from build123d import *

# Parameters (mm, degrees)
SCHIZZO2_W                 = 24
SCHIZZO2_H                 = 35
BASESUPPORTO_DEPTH         = 5
SCHIZZO3_R                 = 8
APPOGGIOALLONGHERONE_DEPTH = 31.120590964
SCHIZZO4_W                 = 5
SCHIZZO4_H                 = 3
FORIFASCETTE_DEPTH         = 22.800229357


with BuildPart() as part:
    # Schizzo2 → BaseSupporto (new body)
    with BuildSketch(Plane(origin=(0, 0, 0), x_dir=(1, 0, 0), z_dir=(0, 1, 0))):
        Rectangle(SCHIZZO2_W, SCHIZZO2_H)
    extrude(amount=BASESUPPORTO_DEPTH)

    # Schizzo3 → AppoggioAlLongherone (cut, through all)
    with BuildSketch(Plane.ZY.offset(12)):
        with Locations((-25.099342077, 2.5)):
            Circle(SCHIZZO3_R)
    extrude(amount=-APPOGGIOALLONGHERONE_DEPTH, mode=Mode.SUBTRACT)

    # Schizzo4 → ForiFascette (cut, through all)
    with BuildSketch(Plane(origin=(0, 5, 0), x_dir=(1, 0, 0), z_dir=(0, 1, 0))):
        with Locations((-6, 14)):
            Rectangle(SCHIZZO4_W, SCHIZZO4_H)
        with Locations((6, 14)):
            Rectangle(SCHIZZO4_W, SCHIZZO4_H)
    extrude(amount=-FORIFASCETTE_DEPTH, mode=Mode.SUBTRACT)


solid = part.part
Source: CAD feature listing. Evaluate the final solid. Frame: model axes, mm. A direction names the side the tool comes from. Give positions to 0.01 mm unless a question says otherwise; leave off trailing zeros. Order: outer loops, then holes, each group sorted by start corner. A loop starts at its lowest first (then second) coordinate and runs counter-clockwise, first axis right, second up. Notation, with made-up numbers: (-38.5, -3.75) -> (4.5, -3.75) arc R8 cw to (4.5, 0.25) -> close; hole circle Ø11 at (-22, 87.5). An arc over 180 degrees is marked (long way). Write item = value, one per line.
Q1. Cut plane A-A, the plane x = 7. Output: boundary loops of the cut face in (y, z).
Data:
outline = (0, -17.5) arc R8 cw to (5, -17.5) -> (5, -15.5) -> (0, -15.5) -> close; (0, -12.5) -> (5, -12.5) -> (5, 17.5) -> (0, 17.5) -> close
Q2. Cut plane B-B, the plane z = -15. Output: boundary loops of the cut face in (x, y).
Data:
outline = (-12, 0) -> (-8.5, 0) -> (-8.5, 5) -> (-12, 5) -> close; (-3.5, 0) -> (3.5, 0) -> (3.5, 5) -> (-3.5, 5) -> close; (8.5, 0) -> (12, 0) -> (12, 5) -> (8.5, 5) -> close
Q3. Set-up query: faces 1 (the face through (-6, 3, -15.5)), 2 (the face through (-0.2, 2.5, -17.1)). Return all of +Z, -Z, +X, -X, +Y, -Y with unobstructed straight access to the full face (end or side cutting, diameter ignored); none if empty.
Data:
face_1 = +Y, -Y
face_2 = -Z, +X, -X
Q4. Cut plane C-C, the plane y = 1.25. Output: boundary loops of the cut face in (x, z).
Data:
outline = (-12, -17.2) -> (12, -17.2) -> (12, 17.5) -> (-12, 17.5) -> close; hole (-8.5, -15.5) -> (-3.5, -15.5) -> (-3.5, -12.5) -> (-8.5, -12.5) -> close; hole (3.5, -15.5) -> (8.5, -15.5) -> (8.5, -12.5) -> (3.5, -12.5) -> close
Q5. Pin query (flat end, axial travel): pin 1 (2.5 mm diameter, centred on x = 5.5, y = 2, fed in from -Z). Return the tip coordinate at first contact, or that it passes through.
Data:
pin_1 = -17.29
Q6. Material intervals for line 1 (Z direction, x = 8, y = 2.45); line 2 (X direction, y = 1.85, z = -15); line 3 (Z direction, x = -4.5, y = 3.75), sorted ascending. Write a range as from..to.
Data:
line_1 = -17.1..-15.5, -12.5..17.5
line_2 = -12..-8.5, -3.5..3.5, 8.5..12
line_3 = -17.2..-15.5, -12.5..17.5
Q7. Pull-direction query (Z, two-part tool) for faces 3 (the face through (0, 5, 0)), 4 (the face through (0, 2, 17.5)), 5 (the face through (6, 3, -15.5)); classes: released by +Z, released by -Z, zero draft, split by the parting line, or undercut.
Data:
face_3 = zero draft
face_4 = released by +Z
face_5 = undercut
